Geometry: final body of the model. Coordinates: model frame, mm. Face numbers are marked on the shaded views. A direction names the side the tool comes from. Coordinates: 2 decimals unless noted, no trailing zeros. Write each loop counter-clockwise with the first axis right and the second up, starting at its lowest first coordinate (ties: lowest second). Pieces come first, ordered by that corner, then holes. Notation, with made-up numbers: (70, 81.25) - (122, 81.25) arc R18 ccw to (122, 113.25) - close; hole circle Ø11 at (-35.75, 4.25). An arc over 180 degrees is marked (long way). Answer as a JSON object with one key per item and string values. Group by question number.
Item 1: Section B-B on y = 11.25. Return loops of the section in (x, z), and give its area (3 significant figures).
Item 2: Line query: line 1 along X through (y, z) = (7, 0); line 2 along Z through (x, y) = (0.75, 5). Output: solid intervals per line, ascending. Write a range as from..to.
Item 3: First-contact query: pin 1 Ø1 at (x, y) = (2, 3.5) entering from -Z; pin 2 Ø4 at (x, y) = (0.5, 14) entering from -Z; pin 3 Ø2 at (y, z) = (9.5, -0.5) entering from +X. Flat tips, straight axial feed; report the tip coordinate or a pass-through.
Item 4: Set-up query: the marked faces 1 and 2. Return all of +Z, -Z, +X, -X, +Y, -Y with unobstructed straight access to the full face (end or side cutting, diameter ignored); none if empty.
Item 5: Section A-A on y = 15.5. Return loops of the section in (x, z).
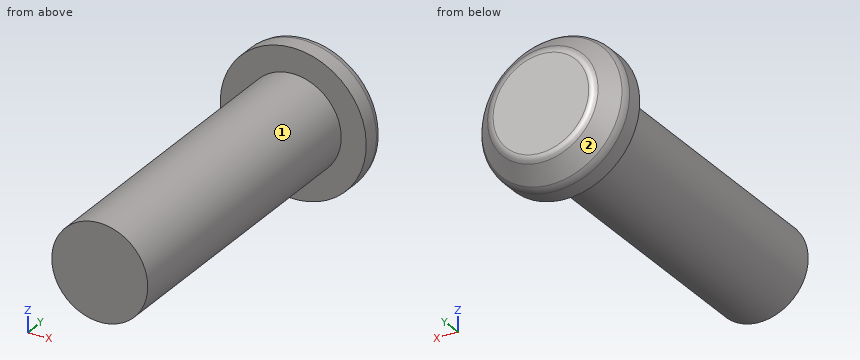
```python
from build123d import *

# Parameters (mm, degrees)
SKETCH1_R           = 2.3
BOSS_EXTRUDE1_DEPTH = 15
SKETCH2_R           = 3.5
BOSS_EXTRUDE2_DEPTH = 2
CHAMFER1_SIZE       = 1
FILLET1_R           = 0.5


with BuildPart() as part:
    # Sketch1 → Boss-Extrude1 (new body)
    with BuildSketch(Plane(origin=(0, 0, 0), x_dir=(1, 0, 0), z_dir=(0, 1, 0))):
        with Locations(Location((0, 0, 0), (0, 0, 270))):
            Circle(SKETCH1_R)
    extrude(amount=BOSS_EXTRUDE1_DEPTH)

    # Sketch2 → Boss-Extrude2 (add)
    with BuildSketch(Plane(origin=(0, 15, 0), x_dir=(1, 0, 0), z_dir=(0, 1, 0))):
        with Locations(Location((0, 0, 0), (0, 0, 270))):
            Circle(SKETCH2_R)
    extrude(amount=BOSS_EXTRUDE2_DEPTH)

    # Chamfer1
    chamfer1_edges = [part.edges().sort_by_distance(p)[0] for p in [
        (0, 17, -3.5),
    ]]
    chamfer(chamfer1_edges, length=CHAMFER1_SIZE)

    # Fillet1
    fillet1_edges = [part.edges().sort_by_distance(p)[0] for p in [
        (0, 17, -2.5),
        (0, 16, -3.5),
    ]]
    fillet(fillet1_edges, radius=FILLET1_R)


solid = part.part
```
Checks:
{
 "1": {"outline": "circle Ø4.6 at (0, 0)", "area": "16.6 mm^2"},
 "2": {"line 1": "-2.3..2.3", "line 2": "-2.17..2.17"},
 "3": {"pin 1": "z = -1.74", "pin 2": "z = -3.5", "pin 3": "x = 2.3"},
 "4": {"face 1": "-Y", "face 2": "+Y"},
 "5": {"outline": "circle Ø7 at (0, 0)"}
}
